Work out the finished part from the listing and answer in its coordinate system (mm). A direction names the side the tool comes from. Coordinates: 2 decimals unless noted, no trailing zeros. Order: outer loops, then holes, each group sorted by start corner. A loop starts at its lowest first (then second) coordinate and runs counter-clockwise, first axis right, second up. Notation, with made-up numbers: (-27, 12) -> (-22, 12) arc R7 cw to (-22, 16) -> close; hole circle Ø2 at (41, 29.25). An arc over 180 degrees is marked (long way). Use one line per item in the form item = value.
from build123d import *

# Parameters (mm, degrees)
F0_W     = 8
F0_H     = 8
F0_R     = 3
F1_DEPTH = 3
F2_W     = 1
F2_H     = 8
F3_DEPTH = 6.45


with BuildPart() as f1:
    # F0 (on Front) → F1 (new body)
    with BuildSketch(Plane.XZ):
        Rectangle(F0_W, F0_H)
        Circle(F0_R, mode=Mode.SUBTRACT)
    extrude(amount=F1_DEPTH)

    # F2 (on face) → F3 (join)
    with BuildSketch(Plane.XZ.offset(3)):
        with Locations((-3.5, 0)):
            Rectangle(F2_W, F2_H)
        with Locations((3.5, 0)):
            Rectangle(F2_W, F2_H)
    extrude(amount=F3_DEPTH)


solid = f1.part
(1) Which of the six approach directions +Z, -Z, +X, -X, +Y, -Y give full straight-line access (tool end or side, diameter ignored) to faces 1 (the flat face through (0, -3, 3.4)), 2 (the flat face through (-0.1, -2.6, 4))?
Data:
face_1 = +Z, -Z, -Y
face_2 = +Z, +X, -X, +Y, -Y
(2) Section C-C on z = -1.75 is taken. Write down the section's boundary in (x, y), plus the area to 3 significant figures.
Data:
outline = (-4, -9.45) -> (-3, -9.45) -> (-3, -3) -> (-2.44, -3) -> (-2.44, 0) -> (-4, 0) -> close; (2.44, -3) -> (3, -3) -> (3, -9.45) -> (4, -9.45) -> (4, 0) -> (2.44, 0) -> close
area = 22.3 mm²
(3) Each of these flat-tipped pins is pushed along its axis until it touches: P1, Ø2, axis at x = -0.5, z = 1.5, coming from the -Y side; P2, Ø3, axis at x = -0.5, z = -2, coming from the -Y side. Where does it stop, or does it pass through?
Data:
P1 = through
P2 = -3
(4) Section B-B on x = 0 is taken. Write down the section's boundary in (y, z), plus the area to 3 significant figures.
Data:
outline = (-3, -4) -> (0, -4) -> (0, -3) -> (-3, -3) -> close; (-3, 3) -> (0, 3) -> (0, 4) -> (-3, 4) -> close
area = 6.00 mm²
(5) Section A-A on y = -3.5 is taken. Write down the section's boundary in (x, z), plus the area to 3 significant figures.
Data:
outline = (-4, -4) -> (-3, -4) -> (-3, 4) -> (-4, 4) -> close; (3, -4) -> (4, -4) -> (4, 4) -> (3, 4) -> close
area = 16.0 mm²
(6) Straight lines are drawn through the part: line 1 along Z through (x, y) = (0, -1); line 2 along X through (y, z) = (-2.25, 1.25). For each, find the intervals that lie inside material, in ascending order.
Data:
line_1 = -4 to -3, 3 to 4
line_2 = -4 to -2.73, 2.73 to 4
(7) Section D-D on y = -0.75 is taken. Write down the section's boundary in (x, z), plus the area to 3 significant figures.
Data:
outline = (-4, -4) -> (4, -4) -> (4, 4) -> (-4, 4) -> close; hole circle Ø6 at (0, 0)
area = 35.7 mm²
(8) The mould has two halves that part along X. Classify faces 3 (the flat face through (4, -5, 0)), 4 (the flat face through (-3, -6, 0)), 5 (the flat face through (3, -6, 0)), 6 (the flat face through (3.5, -9.45, 0.1)): released by +X, released by -X, zero draft, split by the parting line, or undercut.
Data:
face_3 = released by +X
face_4 = undercut
face_5 = undercut
face_6 = zero draft
